Could you check a few things on this model? Use its own coordinates, in mm. Face numbers are marked on the shaded views. A direction names the side the tool comes from. Coordinates: 2 decimals unless noted, no trailing zeros. Loops run counter-clockwise (first coordinate to the right, second up) from the corner with the lowest first, then second, coordinate; pieces in that order, holes last.
Autodesk Inventor part; units mm, degrees
ref_plane "YZ Plane" through (0, 0, 0) normal (1, 0, 0) x (0, 1, 0)
ref_plane "XZ Plane" through (0, 0, 0) normal (0, 1, 0) x (-1, 0, 0)
ref_plane "XY Plane" through (0, 0, 0) normal (0, 0, 1) x (1, 0, 0)
ref_plane "Arbeitsebene3" through (60, 0, -82.935) normal (0, 0, 1) x (1, 0, 0)
sketch "Skizze13" plane through (60, 0, -82.935) normal (0, 0, 1) x (1, 0, 0)
  line L0 (-37.4166, 8.45) -> (-37.4166, 59.55)
  ellipse E0 centre (23.8014, -114.2521) end of major axis (147.0034, -54.0467) minor radius 137.1256 (-36.404, 8.95) -> (-37.4166, 8.45) ccw
  line L1 (-36.404, 8.95) -> (36.404, 8.95)
  ellipse E1 centre (-23.8014, -114.2521) end of major axis (98.9007, -175.47) minor radius 137.1256 (37.4166, 8.45) -> (36.404, 8.95) ccw
  line L2 (37.4166, 59.55) -> (37.4166, 8.45)
  ellipse E2 centre (-23.8014, 182.2521) end of major axis (-147.0034, 122.0467) minor radius 137.1256 (36.404, 59.05) -> (37.4166, 59.55) ccw
  line L3 (36.404, 59.05) -> (-36.404, 59.05)
  ellipse E3 centre (23.8014, 182.2521) end of major axis (-98.9007, 243.47) minor radius 137.1256 (-37.4166, 59.55) -> (-36.404, 59.05) ccw
  arc A0 (11.7926, 47.5991) -> (-11.7926, 47.5991) centre (0, 34) ccw
  arc A1 (13.5991, 45.7926) -> (11.7926, 47.5991) centre (15, 49) ccw
  arc A2 (13.5991, 22.2074) -> (13.5991, 45.7926) centre (0, 34) ccw
  arc A3 (11.7926, 20.4009) -> (13.5991, 22.2074) centre (15, 19) ccw
  arc A4 (-11.7926, 20.4009) -> (11.7926, 20.4009) centre (0, 34) ccw
  arc A5 (-13.5991, 22.2074) -> (-11.7926, 20.4009) centre (-15, 19) ccw
  arc A6 (-13.5991, 45.7926) -> (-13.5991, 22.2074) centre (0, 34) ccw
  arc A7 (-11.7926, 47.5991) -> (-13.5991, 45.7926) centre (-15, 49) ccw
  circle A8 centre (19, 15) radius 1.621
  circle A9 centre (19, 53) radius 1.621
  circle A10 centre (-19, 15) radius 1.621
  circle A11 centre (-19, 53) radius 1.621
  circle A12 centre (0, 34) radius 16
  line L4 (-33.4166, 58.05) -> (33.4166, 58.05)
  line L5 (36.4166, 55.05) -> (36.4166, 12.95)
  line L6 (33.4166, 9.95) -> (-33.4166, 9.95)
  line L7 (-36.4166, 12.95) -> (-36.4166, 55.05)
  arc A13 (-33.4166, 58.05) -> (-36.4166, 55.05) centre (-33.4166, 55.05) ccw
  arc A14 (-36.4166, 12.95) -> (-33.4166, 9.95) centre (-33.4166, 12.95) ccw
  arc A15 (33.4166, 9.95) -> (36.4166, 12.95) centre (33.4166, 12.95) ccw
  arc A16 (36.4166, 55.05) -> (33.4166, 58.05) centre (33.4166, 55.05) ccw
  point P0 (-60, 0)
  dimension "d147" = 32
  dimension "d148" = 1
  dimension "d149" = 3
extrude "Extrusion11" add sketch "Skizze13" along normal blind 8 contours A1 A2 A3 A4 A5 A6 A7 A0 | L4 A16 L5 A15 L6 A14 L7 A13
sketch "Skizze14" plane through (60, 0, -74.935) normal (0, 0, 1) x (1, 0, 0)
  point P0 (-60, 0)
sketch "Skizze15" plane through (60, 0, -74.935) normal (0, 0, 1) x (1, 0, 0)
  line L0 (-33.541, 7.75) -> (-33.541, 50.25)
  line L1 (-33.4166, 9.95) -> (33.4166, 9.95)
  arc A0 (33.4166, 9.95) -> (36.4166, 12.95) centre (33.4166, 12.95) ccw
  line L2 (36.4166, 12.95) -> (36.4166, 55.05)
  arc A1 (36.4166, 55.05) -> (33.4166, 58.05) centre (33.4166, 55.05) ccw
  line L3 (33.4166, 58.05) -> (-33.4166, 58.05)
  arc A2 (-33.4166, 58.05) -> (-36.4166, 55.05) centre (-33.4166, 55.05) ccw
  line L4 (-36.4166, 55.05) -> (-36.4166, 12.95)
  arc A3 (-36.4166, 12.95) -> (-33.4166, 9.95) centre (-33.4166, 12.95) ccw
  circle A4 centre (0, 34) radius 16
  circle A5 centre (-19, 53) radius 1.621
  circle A6 centre (-19, 15) radius 1.621
  circle A7 centre (19, 53) radius 1.621
  circle A8 centre (19, 15) radius 1.621
  line L5 (-77.5, 76.5) -> (77.5, 76.5)
  line L6 (-66, 79) -> (-60, 79)
  line L7 (66, -21) -> (66, 79)
  line L8 (-66, 79) -> (-66, -21)
  line L9 (-77.5, 107.3475) -> (77.5, 107.3475)
  line L10 (-33.4166, 9.95) -> (33.4166, 9.95)
  arc A9 (33.4166, 9.95) -> (36.4166, 12.95) centre (33.4166, 12.95) ccw
  line L11 (36.4166, 12.95) -> (36.4166, 55.05)
  arc A10 (36.4166, 55.05) -> (33.4166, 58.05) centre (33.4166, 55.05) ccw
  line L12 (33.4166, 58.05) -> (-33.4166, 58.05)
  arc A11 (-33.4166, 58.05) -> (-36.4166, 55.05) centre (-33.4166, 55.05) ccw
  line L13 (-36.4166, 55.05) -> (-36.4166, 12.95)
  arc A12 (-36.4166, 12.95) -> (-33.4166, 9.95) centre (-33.4166, 12.95) ccw
  circle A13 centre (0, 34) radius 16
  circle A14 centre (-19, 53) radius 1.621
  circle A15 centre (-19, 15) radius 1.621
  circle A16 centre (19, 53) radius 1.621
  circle A17 centre (19, 15) radius 1.621
  line L14 (-33.4166, 55.05) -> (33.4166, 55.05)
  line L15 (33.4166, 55.05) -> (33.4166, 12.95)
  line L16 (33.4166, 12.95) -> (-33.4166, 12.95)
  line L17 (-33.4166, 12.95) -> (-33.4166, 55.05)
  line L18 (60, -8) -> (-60, -8)
  line L19 (-60, -8) -> (-60, 76)
  line L20 (-60, 76) -> (60, 76)
  line L21 (60, 76) -> (60, -8)
  line L22 (60, -8) -> (-60, 76) construction
  line L23 (-60, -8) -> (60, 76) construction
  line L24 (-60, -8) -> (60, -8)
  line L25 (60, -8) -> (60, -21)
  line L26 (60, -21) -> (-60, -21)
  line L27 (-60, -21) -> (-60, -8)
  point P0 (-60, 0)
  point P1 (60, -8)
extrude "Extrusion12" add sketch "Skizze15" along normal blind 8 contours A3 L4 A2 L3 A1 L2 A0 L1 | L25 L26 L27 L18 | L18 L19 L20 L21
chamfer "Fasen1" distance 3 angle 45 4 edges at (93.4166, 34, -74.935) (60, 12.95, -74.935) (26.5834, 34, -74.935) (60, 55.05, -74.935)
sketch "Skizze16" plane through (60, 0, -66.935) normal (0, 0, 1) x (1, 0, 0)
  line L0 (60, 76) -> (-60, 76)
  line L1 (-60, 76) -> (-60, -21)
  line L2 (-60, -21) -> (60, -21)
  line L3 (60, -21) -> (60, 76)
  line L4 (-33.4166, 55.05) -> (33.4166, 55.05)
  line L5 (33.4166, 55.05) -> (33.4166, 12.95)
  line L6 (33.4166, 12.95) -> (-33.4166, 12.95)
  line L7 (-33.4166, 12.95) -> (-33.4166, 55.05)
  line L8 (-54, 70) -> (54, 70)
  line L9 (54, 70) -> (54, -15)
  line L10 (54, -15) -> (-54, -15)
  line L11 (-54, -15) -> (-54, 70)
  dimension "d163" = 6
extrude "Extrusion13" add sketch "Skizze16" along normal up to surface (101.4112 mm away) contours L3 L2 L1 L0
fillet "Rundung3" radius 5 4 edges at (0, 76, -20.2294) (120, 76, -20.2294) (0, -21, -20.2294) (120, -21, -20.2294)
sketch "Skizze17" plane through (0, -16, -74.935) normal (-1, 0, 0) x (0, 0, 1)
  circle A0 centre (83.4487, 47.5) radius 1.6
  circle A1 centre (83.4487, 32.5) radius 1.6
  circle A2 centre (83.4487, 62.5) radius 1.6
  circle A3 centre (83.4487, 17.5) radius 1.6
  circle A4 centre (83.4487, 77.5) radius 1.6
  line L0 (168.1612, 6.4) -> (168.1612, 4)
  line L1 (168.1612, 4) -> (162.6612, 4)
  line L2 (162.6612, 4) -> (162.6612, 6.4)
  line L3 (162.6612, 6.4) -> (168.1612, 6.4)
  line L4 (128.1612, 6.4) -> (128.1612, 4)
  line L5 (128.1612, 4) -> (122.6612, 4)
  line L6 (122.6612, 4) -> (122.6612, 6.4)
  line L7 (122.6612, 6.4) -> (128.1612, 6.4)
  line L8 (170.6987, 83.6) -> (170.6987, 86)
  line L9 (170.6987, 86) -> (176.1987, 86)
  line L10 (176.1987, 86) -> (176.1987, 83.6)
  line L11 (176.1987, 83.6) -> (170.6987, 83.6)
  line L12 (96.1987, 86) -> (96.1987, 83.6)
  line L13 (96.1987, 83.6) -> (90.6987, 83.6)
  line L14 (90.6987, 83.6) -> (90.6987, 86)
  line L15 (90.6987, 86) -> (96.1987, 86)
  line L16 (193.4487, 87) -> (193.2487, 87)
  line L17 (193.2487, 87) -> (193.2487, 89)
  line L18 (193.4487, 89) -> (193.4487, 91.1929)
  line L19 (190.5112, 89) -> (180.3112, 89)
  line L20 (180.3112, 89) -> (188.3487, 95)
  line L21 (188.3487, 95) -> (178.5487, 95)
  line L22 (178.5487, 95) -> (170.5112, 89)
  line L23 (170.5112, 89) -> (160.3112, 89)
  line L24 (160.3112, 89) -> (168.3487, 95)
  line L25 (168.3487, 95) -> (158.5487, 95)
  line L26 (158.5487, 95) -> (150.5112, 89)
  line L27 (150.5112, 89) -> (140.3112, 89)
  line L28 (140.3112, 89) -> (148.3487, 95)
  line L29 (148.3487, 95) -> (138.5487, 95)
  line L30 (138.5487, 95) -> (130.5112, 89)
  line L31 (130.5112, 89) -> (120.3112, 89)
  line L32 (120.3112, 89) -> (128.3487, 95)
  line L33 (128.3487, 95) -> (118.5487, 95)
  line L34 (118.5487, 95) -> (110.5112, 89)
  line L35 (110.5112, 89) -> (100.3112, 89)
  line L36 (100.3112, 89) -> (108.3487, 95)
  line L37 (108.3487, 95) -> (98.5487, 95)
  line L38 (98.5487, 95) -> (90.5112, 89)
  line L39 (90.5112, 89) -> (80.3112, 89)
  line L40 (80.3112, 89) -> (88.3487, 95)
  line L41 (88.3487, 95) -> (78.4487, 95)
  line L42 (120.3112, -5) -> (120.3112, 1)
  line L43 (120.3112, 1) -> (130.5112, 1)
  line L44 (130.5112, 1) -> (130.5112, -5)
  line L45 (140.3112, -5) -> (140.3112, 1)
  line L46 (140.3112, 1) -> (150.5112, 1)
  line L47 (150.5112, 1) -> (150.5112, -5)
  line L48 (160.3112, -5) -> (160.3112, 1)
  line L49 (160.3112, 1) -> (170.5112, 1)
  line L50 (170.5112, 1) -> (170.5112, -5)
  line L51 (180.4112, -5) -> (180.4112, 1)
  line L52 (180.4112, 1) -> (185.4112, 1)
  line L53 (193.2487, 89) -> (193.4487, 89)
  line L54 (193.4487, 91.1929) -> (190.5112, 89)
  line L55 (78.4487, 95) -> (78.4487, -5)
  line L56 (78.4487, -5) -> (120.3112, -5)
  line L57 (130.5112, -5) -> (140.3112, -5)
  line L58 (150.5112, -5) -> (160.3112, -5)
  line L59 (170.5112, -5) -> (180.4112, -5)
  line L60 (185.4112, 1) -> (185.4112, -5)
  line L61 (185.4112, -5) -> (193.4487, -5)
  line L62 (193.4487, -5) -> (193.4487, 87)
  point P0 (74.935, 16)
hole "Bohrung3" at (0, 61.5, 8.5137) at (0, 46.5, 8.5137) at (0, 31.5, 8.5137) at (0, 16.5, 8.5137) at (0, 1.5, 8.5137) direction (1, 0, 0) diameter 3.2 end through all
properties part number "OpenFrameAdapter"
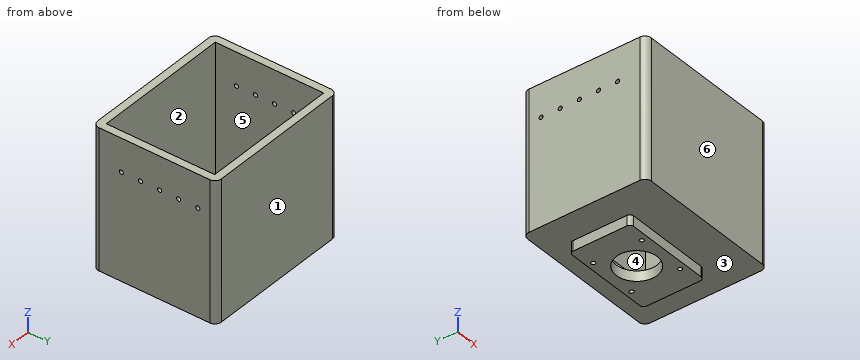
(1) For pin 1 (6.5 mm diameter, centred on y = 33.5, z = -80.5, fed in from +X); pin 2 (8 mm diameter, centred on x = 70.5, y = 53, fed in from +Z) (3 decimals); pin 3 (1.5 mm diameter, centred on x = 35, y = 47.5, fed in from +Z) (3 decimals); pin 4 (19 mm diameter, centred on x = 60, y = 34, fed in from +Z), each with a flat end and sliding along its axis, tell me the tip position at first contact or that it passes through.
Answers:
pin 1: stops at x = 96.42
pin 2: stops at z = -66.935
pin 3: stops at z = -74.935
pin 4: passes through
(2) Imagine slicing it at D-D, the plane y = 31.5. State how many separate pieces and enclosed holes the cut face has, and give its area (3 significant figures).
Answers:
separate pieces: 4
enclosed holes: 0
area: 1,940 mm2
(3) We'd pull the mould along Y, two halves only. Please class the marked faces 3, 4, 5 and 6: +Y half, -Y half, draft (parallel to the pull), parting line (faces both ways), or undercut.
Answers:
face 3: draft
face 4: undercut
face 5: undercut
face 6: -Y half
(4) I need wall thicknesses on probe 1 along Y at (x, z) = (79, -78.5); probe 2 along X at (y, z) = (53, -78); probe 3 along X at (y, z) = (32, 19). Which ranges of each line are inside material? Lowest first, please.
Answers:
probe 1: y = 9.95 to 13.38, 16.62 to 51.38, 54.62 to 58.05
probe 2: x = 23.58 to 39.38, 42.62 to 77.38, 80.62 to 96.42
probe 3: x = 0 to 6, 114 to 120
(5) Imagine slicing it at B-B, the plane z = -17.5. Write out the boundary of the cut face in (x, y), and give its area (3 significant figures).
Answers:
outline: (0, -16) arc R5 ccw to (5, -21) - (115, -21) arc R5 ccw to (120, -16) - (120, 71) arc R5 ccw to (115, 76) - (5, 76) arc R5 ccw to (0, 71) - close; hole (6, -15) - (114, -15) - (114, 70) - (6, 70) - close
area: 2,440 mm2
(6) Imagine slicing it at A-A, the plane y = 1.5. Write out the boundary of the cut face in (x, z) (3 decimals).
Answers:
outline: (0, -74.935) - (120, -74.935) - (120, 6.914) - (114, 6.914) - (114, -66.935) - (6, -66.935) - (6, 6.914) - (0, 6.914) - close; (0, 10.114) - (6, 10.114) - (6, 34.476) - (0, 34.476) - close; (114, 10.114) - (120, 10.114) - (120, 34.476) - (114, 34.476) - close
(7) Which directions (+Z, -Z, +X, -X, +Y, -Y) give clear straight access to the entire face, cutting with the end or side of a thin tool? Please do the marked faces 1 and 2.
Answers:
face 1: +Z, -Z, +X, -X, +Y
face 2: +Z
